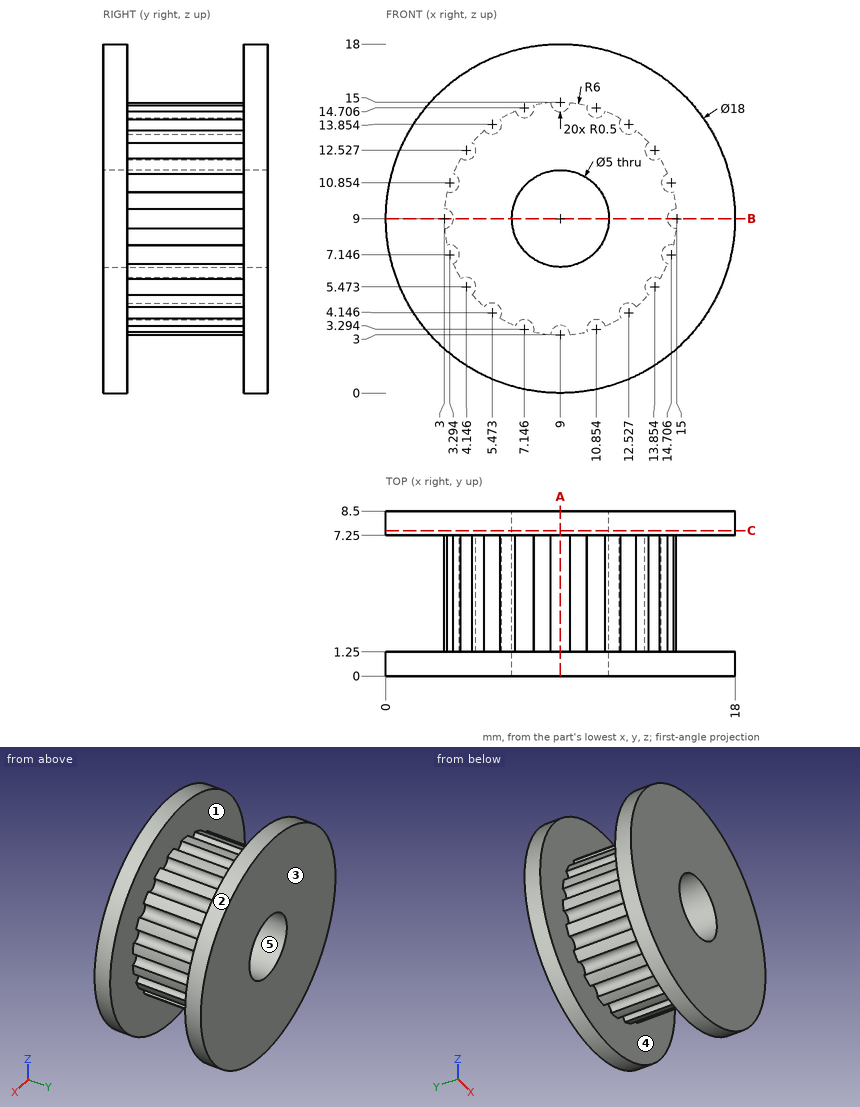
Source: three-view drawing plus pictorial views. Frame: mm from the lowest corner of the part. A direction names the side the tool comes from. Round coordinates to 2 decimals unless told otherwise and drop trailing zeros. Write each loop counter-clockwise with the first axis right and the second up, starting at its lowest first coordinate (ties: lowest second). Pieces come first, ordered by that corner, then holes. Notation, with made-up numbers: (52.25, -16) -> (108.25, -16) arc R19 cw to (108.25, -11) -> close; hole circle Ø7 at (80.5, -12.5). An arc over 180 degrees is marked (long way). Return JSON: item names as keys, results as strings.
Q1. Mould query, pull axis Y, two halves, no side actions, for the marked faces 1, 2 and 3. Classes: +Y half, -Y half, draft (parallel to the pull), parting line (faces both ways), or undercut.
From the geometry:
{"face 1": "undercut", "face 2": "draft", "face 3": "+Y half"}
Q2. Section A-A on x = 9. Return the cut outline in (y, z).
From the geometry:
{"outline": "(0, 0) -> (1.25, 0) -> (1.25, 3.5) -> (7.25, 3.5) -> (7.25, 0) -> (8.5, 0) -> (8.5, 6.5) -> (0, 6.5) -> close; (0, 11.5) -> (8.5, 11.5) -> (8.5, 18) -> (7.25, 18) -> (7.25, 14.5) -> (1.25, 14.5) -> (1.25, 18) -> (0, 18) -> close"}
Q3. Section B-B on z = 9. Return the cut outline in (x, y).
From the geometry:
{"outline": "(0, 0) -> (6.5, 0) -> (6.5, 8.5) -> (0, 8.5) -> (0, 7.25) -> (3.5, 7.25) -> (3.5, 1.25) -> (0, 1.25) -> close; (11.5, 0) -> (18, 0) -> (18, 1.25) -> (14.5, 1.25) -> (14.5, 7.25) -> (18, 7.25) -> (18, 8.5) -> (11.5, 8.5) -> close"}
Q4. First-contact query: pin 1 Ø8 at (x, z) = (8.5, 10) entering from +Y; pin 2 Ø5 at (y, z) = (5, 3.5) entering from +X (1 decimal); pin 3 Ø3 at (y, z) = (1.5, 6) entering from -X. Flat tips, straight axial feed; report the tip coordinate or a pass-through.
From the geometry:
{"pin 1": "y = 8.5", "pin 2": "x = 16.8", "pin 3": "x = 0.13"}
Q5. Ray query, line 1 (Y direction, x = 4.25, z = 3.25); line 2 (X direction, y = 3.5, z = 7); line 3 (Z direction, x = 9.25, y = 4.75). Return the intervals inside material, ascending.
From the geometry:
{"line 1": "0 to 1.25, 7.25 to 8.5", "line 2": "3.77 to 7.5, 10.5 to 14.23", "line 3": "3.43 to 6.51, 11.49 to 14.57"}
Q6. Section C-C on y = 7.5. Return the cut outline in (x, z), and give its area (3 significant figures).
From the geometry:
{"outline": "circle Ø18 at (9, 9); hole circle Ø5 at (9, 9)", "area": "235 mm2"}
Q7. Set-up query: the marked faces 4 and 5. Return all of +Z, -Z, +X, -X, +Y, -Y with unobstructed straight access to the full face (end or side cutting, diameter ignored); none if empty.
From the geometry:
{"face 4": "none", "face 5": "+Y, -Y"}
